from build123d import *

# Parameters (mm, degrees)
F0_W     = 210
F0_H     = 225
F1_DEPTH = 25
F3_DEPTH = 25


with BuildPart() as f1:
    # F0 (on Top) → F1 (new body)
    with BuildSketch(Plane.XY):
        Rectangle(F0_W, F0_H)
    extrude(amount=F1_DEPTH)

    # F2 (on face) → F3 (join)
    with BuildSketch(Plane.XY.offset(25)):
        with BuildLine():
            Line((-71, -32.5), (-71, -112.5))
            Line((-71, -112.5), (-56, -112.5))
            Line((-56, -112.5), (-56, -46.481817))
            ThreePointArc((-56, -46.481817), (7.488853, -14.988853), (38.981817, 48.5))
            Line((38.981817, 48.5), (105, 48.5))
            Line((105, 48.5), (105, 63.5))
            Line((105, 63.5), (25, 63.5))
            ThreePointArc((25, 63.5), (-3.117749, -4.382251), (-71, -32.5))
        make_face()
    extrude(amount=F3_DEPTH)


solid = f1.part
Verification items for the finished model (mm, model axes). A direction names the side the tool comes from. Give positions to 0.01 mm unless a question says otherwise; leave off trailing zeros. Write each loop counter-clockwise with the first axis right and the second up, starting at its lowest first coordinate (ties: lowest second). Pieces come first, ordered by that corner, then holes. Notation, with made-up numbers: M 13.25,-6.5 L 37.25,-6.5 A30 ccw 37.25,32.5 Z; hole C 89,28 d6. An arc over 180 degrees is marked long. Put each result on its own line as item: value. Start each with the question number.
1. Section check C-C (y = 57). Record the cut outline in (x, z), and give its area (3 significant figures).
2. Draft check along Y on faces 1 (the face through (105, -2, 14)), 2 (the face through (-1, -112.5, 14)), 3 (the face through (66, 63.5, 37)). Enter one of: +Y half, -Y half, draft (parallel to the pull), parting line (faces both ways), or undercut.
3. Set-up check for faces 4 (the face through (-71, -72, 37)), 5 (the face through (-3, -5, 50)), 6 (the face through (-105, -2, 12)), 7 (the face through (-56, -80, 37)), 8 (the face through (-25, 27, 25)): record each of +Z, -Z, +X, -X, +Y, -Y from which the full face is reachable in a straight line by a thin tool's end or side.
4. Section check A-A (x = 90.5). Record the cut outline in (y, z).
5. Section check D-D (x = -88.5). Record the cut outline in (y, z), and give its area (4 significant figures).
6. Go/stop test with flat-tipped pins: pin 1 Ø10 at (x, y) = (52.5, -80.5) entering from -Z; pin 2 Ø12 at (x, y) = (53.5, -7) entering from +Z; pin 3 Ø12.5 at (x, z) = (70.5, 37) entering from -Y; pin 4 Ø7.5 at (y, z) = (-79, 38.5) entering from -X. Record where each tip stops, or that it passes through.
7. Section check B-B (z = 35). Record the cut outline in (x, y), and give its area (3 significant figures).
8. Scan lines: line 1 along Z through (x, y) = (42.5, -46); line 2 along Y through (x, z) = (93.5, 29); line 3 along X through (y, z) = (-88, 35). Record each from-to range of solid material in increasing order. Write a range as [from, to].
Answer list:
1. outline: M -105,0 L 105,0 L 105,50 L 24.78,50 L 24.78,25 L -105,25 Z
1. area: 7,260 mm2
2. face 1: draft
2. face 2: -Y half
2. face 3: +Y half
3. face 4: +Z, -X, +Y, -Y
3. face 5: +Z, +X, -X, +Y, -Y
3. face 6: +Z, -Z, -X, +Y, -Y
3. face 7: +Z, +X, -Y
3. face 8: +Z, -X, +Y
4. outline: M -112.5,0 L 112.5,0 L 112.5,25 L 63.5,25 L 63.5,50 L 48.5,50 L 48.5,25 L -112.5,25 Z
5. outline: M -112.5,0 L 112.5,0 L 112.5,25 L -112.5,25 Z
5. area: 5,625 mm2
6. pin 1: z = 0
6. pin 2: z = 25
6. pin 3: y = 48.5
6. pin 4: x = -71
7. outline: M -71,-112.5 L -56,-112.5 L -56,-46.48 A111 ccw 38.98,48.5 L 105,48.5 L 105,63.5 L 25,63.5 A96 cw -71,-32.5 Z
7. area: 4,400 mm2
8. line 1: [0, 25]
8. line 2: [48.5, 63.5]
8. line 3: [-71, -56]
